Part print with two shaded views. Sizes in mm from the minimum x, y, z corner. A direction names the side the tool comes from. Round coordinates to 2 decimals unless told otherwise and drop trailing zeros. Write each loop counter-clockwise with the first axis right and the second up, starting at its lowest first coordinate (ties: lowest second). Pieces come first, ordered by that corner, then holes. Notation, with made-up numbers: (43, 69) - (51, 69) arc R33 cw to (51, 108) - close; hole circle Ø9 at (29.5, 56.5). An arc over 180 degrees is marked (long way). Use one line per item in the form item = value. Start each with the question number.
Item 1: Band-saw the part on C-C, the plane z = 3.2. List the corners of the cut face in (x, y).
Item 2: Drill centre lines: L1, parallel to Y at x = 2.65, z = 2.6; L2, parallel to Y at x = 1.45, z = 3.8; L3, parallel to X at y = 9.5, z = 2.75 (1 decimal). Where is each one in solid material? Low to high.
Item 3: Band-saw the part on D-D, the plane y = 4.5. List the corners of the cut face in (x, z).
Item 4: Tool access for the marked faces 1 and 2: list every direction of +Z, -Z, +X, -X, +Y, -Y with a clear straight run to the whole face (end or side of a thin tool).
Item 5: Band-saw the part on B-B, the plane y = 10. List the corners of the cut face in (x, z) (1 decimal).
Item 6: Band-saw the part on A-A, the plane x = 2.9. List the corners of the cut face in (y, z).
Item 7: Pull direction X, two halves, no side cores. Call the marked faces 3, 4 and 5: +X half, -X half, draft (parallel to the pull), parting line (faces both ways), or undercut.
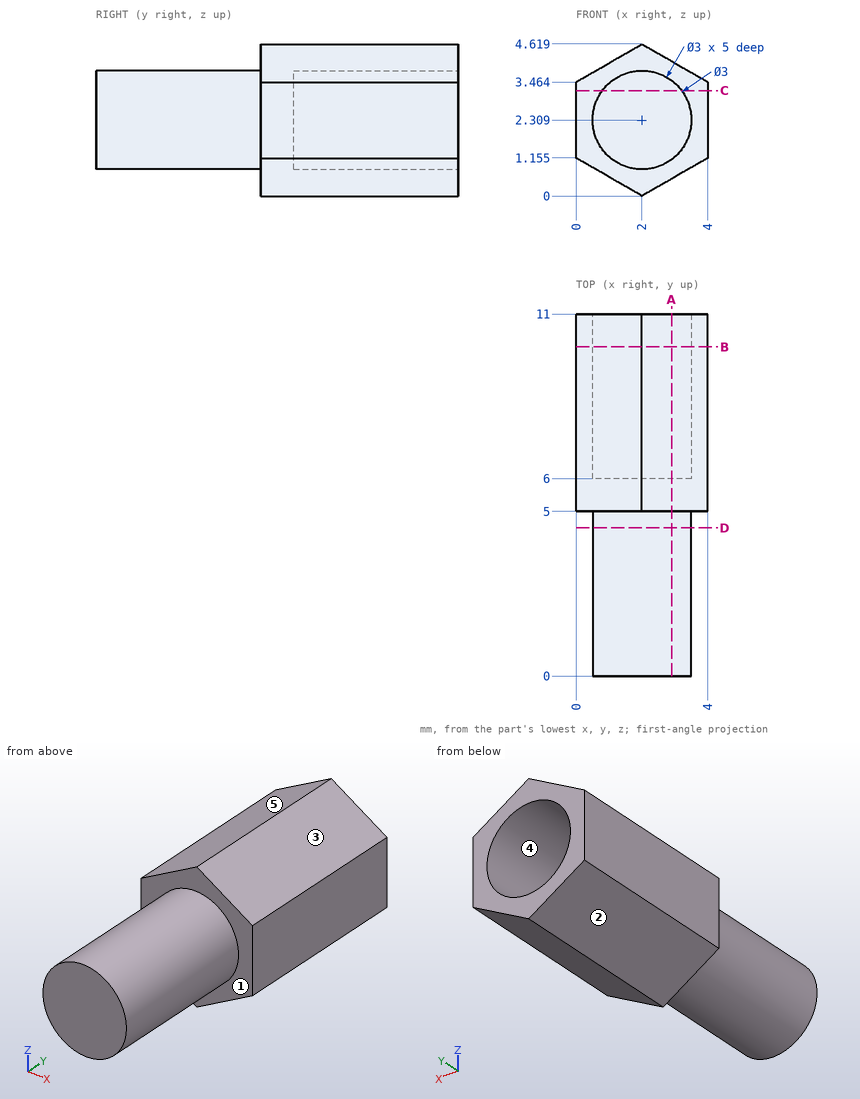
Determined:
q1.outline = (0, 5) - (0.79, 5) - (0.79, 0) - (3.21, 0) - (3.21, 5) - (4, 5) - (4, 11) - (3.21, 11) - (3.21, 6) - (0.79, 6) - (0.79, 11) - (0, 11) - close
q2.L1 = 0 to 6
q2.L2 = 5 to 11
q2.L3 = 0 to 0.6, 3.4 to 4
q3.outline = circle Ø3 at (2, 2.31)
q4.face_1 = -Y
q4.face_2 = -Z, -X, +Y, -Y
q5.outline = (0, 1.2) - (2, 0) - (4, 1.2) - (4, 3.5) - (2, 4.6) - (0, 3.5) - close; hole circle Ø3 at (2, 2.3)
q6.outline = (0, 1.11) - (5, 1.11) - (5, 0.52) - (11, 0.52) - (11, 1.11) - (6, 1.11) - (6, 3.51) - (11, 3.51) - (11, 4.1) - (5, 4.1) - (5, 3.51) - (0, 3.51) - close
q7.face_3 = +X half
q7.face_4 = undercut
q7.face_5 = -X half
